Verification items for the finished model (mm, model axes). Face numbers are marked on the shaded views. A direction names the side the tool comes from. Coordinates: 2 decimals unless noted, no trailing zeros. Order: outer loops, then holes, each group sorted by start corner. A loop starts at its lowest first (then second) coordinate and runs counter-clockwise, first axis right, second up.
Q1. Set-up check for the marked faces 4, 5, 6 and 7: record each of +Z, -Z, +X, -X, +Y, -Y from which the full face is reachable in a straight line by a thin tool's end or side.
Q2. Cross-section at A-A, the plane x = 4. Record the boundary of the cut face in (y, z).
Q3. Draft check along Z on the marked faces 1, 2 and 3. Enter one of: pulls with the +Z half, pulls with the -Z half, needs draft (parallel to the pull), parting line crosses it, or undercut.
Q4. Cross-section at C-C, the plane y = -25. Record the boundary of the cut face in (x, z).
Q5. Depth check by flat-ended pin: P1, Ø0.5, axis at x = 12, z = 16, coming from the +Y side; P2, Ø5, axis at y = -18.5, z = -11, coming from the +X side. Enter the tip coordinate at first touch or a pass-through.
Q6. Cross-section at B-B, the plane y = -21. Record the boundary of the cut face in (x, z).
Q7. Cross-section at D-D, the plane z = 1.5. Record the boundary of the cut face in (x, y), and give its area (3 significant figures).
Q8. Thickness scan on line 1 (Z direction, x = -16, y = -1.4); line 2 (Z direction, x = 4, y = -0.9); line 3 (X direction, y = -0.6, z = -13). Record the ranges inside material, lowest first.
from build123d import *

# Parameters (mm, degrees)
SKETCH_W                 = 35
SKETCH_H                 = 33
PAD_DEPTH                = 20
SKETCH001_W              = 7
SKETCH001_H              = 12
POCKET_DEPTH             = 10
SKETCH004_W              = 36
SKETCH004_H              = 2
POCKET002_DEPTH          = 18.001
POCKET002_DEPTH_BACK     = 15.001
SKETCH002_W              = 5
SKETCH002_H              = 10
PAD001_DEPTH             = 20
SKETCH003_R              = 1.2
POCKET001_DEPTH          = 22.001
POCKET003_DEPTH          = 6
CHAMFER_SIZE             = 5.9
CHAMFER001_SIZE          = 1.6
CHAMFER002_SIZE          = 2
FILLET_R                 = 3
SKETCH010_R              = 2.8
POCKET006_DEPTH          = 2
LINEARPATTERN_COUNT      = 4
LINEARPATTERN_PITCH      = 10
SKETCH012_R              = 3.5
POCKET007_DEPTH          = 8
SKETCH013_W              = 3.523392
SKETCH013_H              = 1.7
SKETCH013_W_2            = 3.89822
PAD003_DEPTH             = 0.4
POCKET008_DEPTH          = 6
CLONE001_PLACEMENT_ANGLE = 90


with BuildPart() as sphere:
    # Sphere → Sphere (revolve)
    with BuildSketch(Plane(origin=(-18, 7, 10), x_dir=(1, 0, 0), z_dir=(0, -1, 0))):
        with BuildLine():
            ThreePointArc((0, -8.3), (8.3, 0), (0, 8.3))
            Line((0, 8.3), (0, -8.3))
        make_face()
    revolve(axis=Axis((-18, 7, 10), (0, 0, 1)))


with BuildPart() as out_socket:
    # Sketch → Pad (new body)
    with BuildSketch(Plane.XY):
        with Locations((-4.5, 1.5)):
            Rectangle(SKETCH_W, SKETCH_H)
    extrude(amount=PAD_DEPTH)

    # Sketch001 (on Face6 of Pad) → Pocket (cut)
    with BuildSketch(Plane.XY.offset(20)):
        with Locations((-17.5, -9)):
            Rectangle(SKETCH001_W, SKETCH001_H)
        with Locations((-4.5, -9)):
            Rectangle(SKETCH001_W, SKETCH001_H)
    extrude(amount=-POCKET_DEPTH, mode=Mode.SUBTRACT)

    # Sketch004 → Pocket002 (cut, two sides)
    with BuildSketch(Plane.XZ) as pocket002_sk:
        with Locations((-7, 10)):
            Rectangle(SKETCH004_W, SKETCH004_H)
    extrude(amount=-POCKET002_DEPTH, mode=Mode.SUBTRACT)
    extrude(pocket002_sk.sketch, amount=POCKET002_DEPTH_BACK, mode=Mode.SUBTRACT)

    # Sketch002 (on Face8 of Pocket002) → Pad001 (join)
    with BuildSketch(Plane.XY.offset(9)):
        with Locations((-17.5, -10)):
            Rectangle(SKETCH002_W, SKETCH002_H)
        with Locations((-4.5, -10)):
            Rectangle(SKETCH002_W, SKETCH002_H)
    extrude(amount=PAD001_DEPTH)

    # Sketch003 → Pocket001 (cut, through all)
    with BuildSketch(Plane.YZ):
        with Locations((-9, 25)):
            Circle(SKETCH003_R)
    extrude(amount=-POCKET001_DEPTH, mode=Mode.SUBTRACT)

    # Sketch005 (on Face4 of Pocket001) → Pocket003 (cut)
    with BuildSketch(Plane.XY.offset(20)):
        Polygon((-6.878414, 11.506697), (-1, -3), (-1, -16.521692), (16.145611, -16.521692), (16.145611, 20.333527), (-18.556482, 20.333527), (-13.204168, 18), align=None)
    extrude(amount=-POCKET003_DEPTH, mode=Mode.SUBTRACT)

    # Chamfer
    chamfer_edges = [out_socket.edges().sort_by_distance(p)[0] for p in [
        (-17.602084, 18, 20),
        (-10.041291, 14.753349, 20),
        (-3.939207, 4.253349, 20),
    ]]
    chamfer(chamfer_edges, length=CHAMFER_SIZE)

    # Chamfer001
    chamfer001_edges = [out_socket.edges().sort_by_distance(p)[0] for p in [
        (-4.5, 18, 0),
        (13, 1.5, 0),
        (-4.5, -15, 0),
        (-22, 1.5, 0),
        (-22, 18, 4.5),
        (-22, -15, 4.5),
        (-22, 18, 12.55),
        (13, 1.5, 14),
        (-0.102084, 18, 14),
    ]]
    chamfer(chamfer001_edges, length=CHAMFER001_SIZE)

    # Chamfer002
    chamfer002_edges = [out_socket.edges().sort_by_distance(p)[0] for p in [
        (-17.5, -15, 29),
        (-4.5, -15, 29),
    ]]
    chamfer(chamfer002_edges, length=CHAMFER002_SIZE)

    # Fillet
    fillet_edges = [out_socket.edges().sort_by_distance(p)[0] for p in [
        (-4.5, -5, 29),
        (-17.5, -5, 29),
    ]]
    fillet(fillet_edges, radius=FILLET_R)

    # Sketch010 → Pocket006 (cut)
    with BuildSketch(Plane.XY):
        with Locations((14, -13)):
            Circle(SKETCH010_R)
        with Locations((4, -13)):
            Circle(SKETCH010_R)
        with Locations((-6, -13)):
            Circle(SKETCH010_R)
        with Locations((-16, -13)):
            Circle(SKETCH010_R)
    pocket006 = extrude(amount=POCKET006_DEPTH, mode=Mode.SUBTRACT)

    # LinearPattern: Pocket006 ×4
    with Locations(*[(0, i * LINEARPATTERN_PITCH, 0) for i in range(1, LINEARPATTERN_COUNT)]):
        add(pocket006, mode=Mode.SUBTRACT)

    # Sketch012 (on Face5 of Pad) → Pocket007 (cut)
    with BuildSketch(Plane(origin=(0, 0, 0), x_dir=(1, 0, 0), z_dir=(0, 0, -1))):
        with Locations((-16, -7)):
            Circle(SKETCH012_R)
    extrude(amount=-POCKET007_DEPTH, mode=Mode.SUBTRACT)

    # Sketch013 (on Face3 of Pad) → Pad003 (join)
    with BuildSketch(Plane.XZ.offset(15)):
        with Locations((-19.82605, 19.15)):
            Rectangle(SKETCH013_W, SKETCH013_H)
        with Locations((-19.451214, 11.85)):
            Rectangle(SKETCH013_W_2, SKETCH013_H)
    extrude(amount=-PAD003_DEPTH)

    # Sketch014 (on Face9 of Pocket) → Pocket008 (cut)
    with BuildSketch(Plane(origin=(-14, 0, 0), x_dir=(0, -1, 0), z_dir=(-1, 0, 0))):
        Polygon((3, 11), (23, 14.52654), (23, 11), align=None)
    extrude(amount=-POCKET008_DEPTH, mode=Mode.SUBTRACT)

    # Cut: cut Sphere
    add(sphere.part, mode=Mode.SUBTRACT)


with BuildPart() as out_socket_1:
    # Clone001 placement: moved
    add(out_socket.part.rotate(Axis((0, 0, 0), (1, 0, 0)), CLONE001_PLACEMENT_ANGLE))


solid = out_socket_1.part
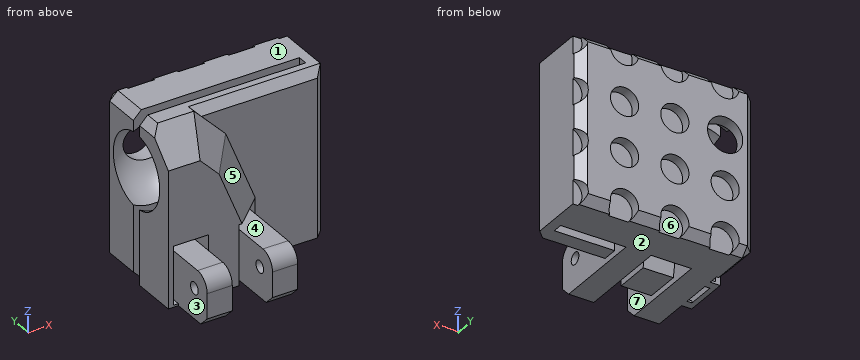
Check values:
1. face 4: -Y
1. face 5: +Z, +X, -Y
1. face 6: +Y
1. face 7: -Z, -Y
2. outline: (-14, -15) - (-11, -15) - (-11, 18) - (-12.4, 18) - (-14, 16.4) - close; (-9, -15) - (-2, -15) - (-2, -10.2) - (0, -10.2) - (0, -5.8) - (-2, -5.8) - (-2, -0.2) - (0, -0.2) - (0, 4.2) - (-2, 4.2) - (-2, 9.8) - (0, 9.8) - (0, 14.2) - (-2, 14.2) - (-2, 18) - (-9, 18) - close
3. face 1: pulls with the +Z half
3. face 2: pulls with the -Z half
3. face 3: undercut
4. outline: (-20, -15) - (-15, -15) - (-15, -10.2) - (-20, -10.2) - close; (-20, -7.8) - (-15, -7.8) - (-15, -5) - (-20, -5) - close; (-7, -15) - (-2, -15) - (-2, -10.2) - (-7, -10.2) - close; (-7, -7.8) - (-2, -7.8) - (-2, -5) - (-7, -5) - close
5. P1: stops at y = -2
5. P2: stops at x = -2
6. outline: (-20, -15) - (-15, -15) - (-15, -5) - (-20, -5) - close; (-7, -15) - (-2, -15) - (-2, -5) - (-7, -5) - close
7. outline: (-22, -20) - (-9.19, -20) - (-2.82, -14.1) - (-2.82, -14) - (11.4, -14) - (13, -12.4) - (13, -1.6) - (11.4, 0) - (-20.4, 0) - (-22, -1.6) - (-22, -5.24) arc R6.22 cw to (-11.86, -9) - (11, -9) - (11, -11) - (-11.86, -11) arc R6.22 cw to (-22, -14.76) - close
7. area: 430 mm2
8. line 1: z = -10.2 to -5.8, -0.2 to 3.5, 10.5 to 14.2
8. line 2: z = -10.2 to -5.8, -0.2 to 4.2, 9.8 to 14.2
8. line 3: x = -21 to -18.8, -13.2 to -8.8, -3.2 to 1.2, 6.8 to 11.2
